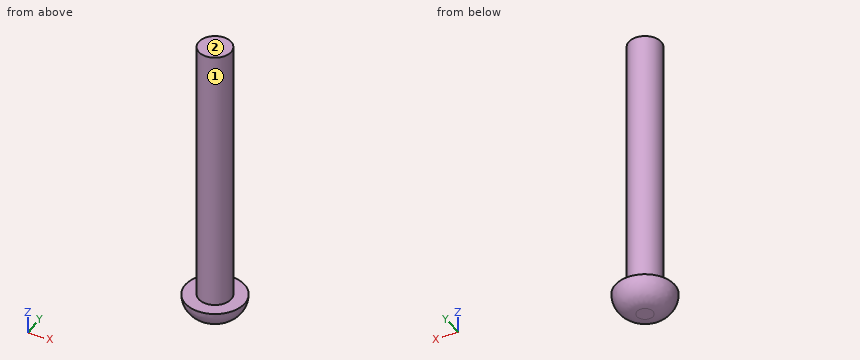
Autodesk Inventor part; units mm, degrees
ref_plane "YZ Plane" through (0, 0, 0) normal (1, 0, 0) x (0, 1, 0)
ref_plane "XZ Plane" through (0, 0, 0) normal (0, 1, 0) x (-1, 0, 0)
ref_plane "XY Plane" through (0, 0, 0) normal (0, 0, 1) x (1, 0, 0)
sketch "スケッチ1" plane through (0, 0, 0) normal (0, 0, 1) x (1, 0, 0)
  circle A0 centre (0, 0) radius 1.5
  dimension "d0" = 3
extrude "押し出し1" add sketch "スケッチ1" along normal blind 25
sketch "スケッチ2" plane through (0, 0, 0) normal (0, 0, -1) x (-1, 0, 0)
  circle A0 centre (0, 0) radius 2.75
  dimension "d3" = 5.5
extrude "押し出し2" add sketch "スケッチ2" along normal blind 2
fillet "フィレット1" radius 2 1 edges at (2.75, 0, -2)
thread "ねじ1"
properties part number "ネジ鍋m3,25" material "鋼、高強度、低合金"
Model file for the job. Use its own axes, mm. Face numbers are marked on the shaded views. A direction names the side the tool comes from. Coordinates: 2 decimals unless noted, no trailing zeros. Order: outer loops, then holes, each group sorted by start corner. A loop starts at its lowest first (then second) coordinate and runs counter-clockwise, first axis right, second up. Notation, with made-up numbers: (-26, 5.5) - (12, 5.5) arc R12 ccw to (12, 15.5) - close; hole circle Ø10 at (68.5, 10). An arc over 180 degrees is marked (long way). Return JSON: item names as keys, results as strings. Group by question number.
1) Flat gauge pins, fed straight in: P1, Ø1.5, axis at y = -0.5, z = 4, coming from the -X side; P2, Ø1.5, axis at x = 2, z = 11, coming from the -Y side; P3, Ø3, axis at x = 0, z = 9, coming from the +Y side. Where does each tip first touch, or does it go through?
2) Tool access for the marked faces 1 and 2: list every direction of +Z, -Z, +X, -X, +Y, -Y with a clear straight run to the whole face (end or side of a thin tool).
3) Probe line 1 (Y direction, x = 0.35, z = 2.5); line 2 (Y direction, x = 0.45, z = 5); line 3 (Z direction, x = -1.65, y = -1.5). List the from-to ranges inside material, lowest first. Write a range as from..to.
4) Saw through at A-A, the plane z = 14. Write the cut outline in (x, y), plus the area to 3 significant figures.
Values found:
{
 "1": {"P1": "stops at x = -1.5", "P2": "stops at y = -0.83", "P3": "stops at y = 1.5"},
 "2": {"face 1": "+Z", "face 2": "+Z, +X, -X, +Y, -Y"},
 "3": {"line 1": "y = -1.46..1.46", "line 2": "y = -1.43..1.43", "line 3": "z = -1.35..0"},
 "4": {"outline": "circle Ø3 at (0, 0)", "area": "7.07 mm²"}
}
